Geometry: see drawing. Coordinates: mm, zero at the bounding-box minimum. A direction names the side the tool comes from. Coordinates: 2 decimals unless noted, no trailing zeros. Loops run counter-clockwise (first coordinate to the right, second up) from the corner with the lowest first, then second, coordinate; pieces in that order, holes last. Notation, with made-up numbers: (74.5, -29.5) - (131.5, -29.5) arc R23 ccw to (131.5, 5.5) - close; hole circle Ø2 at (38.5, 85). An arc over 180 degrees is marked (long way). Write each question's results on one line, items separated by ' | '. Start each with the question number.
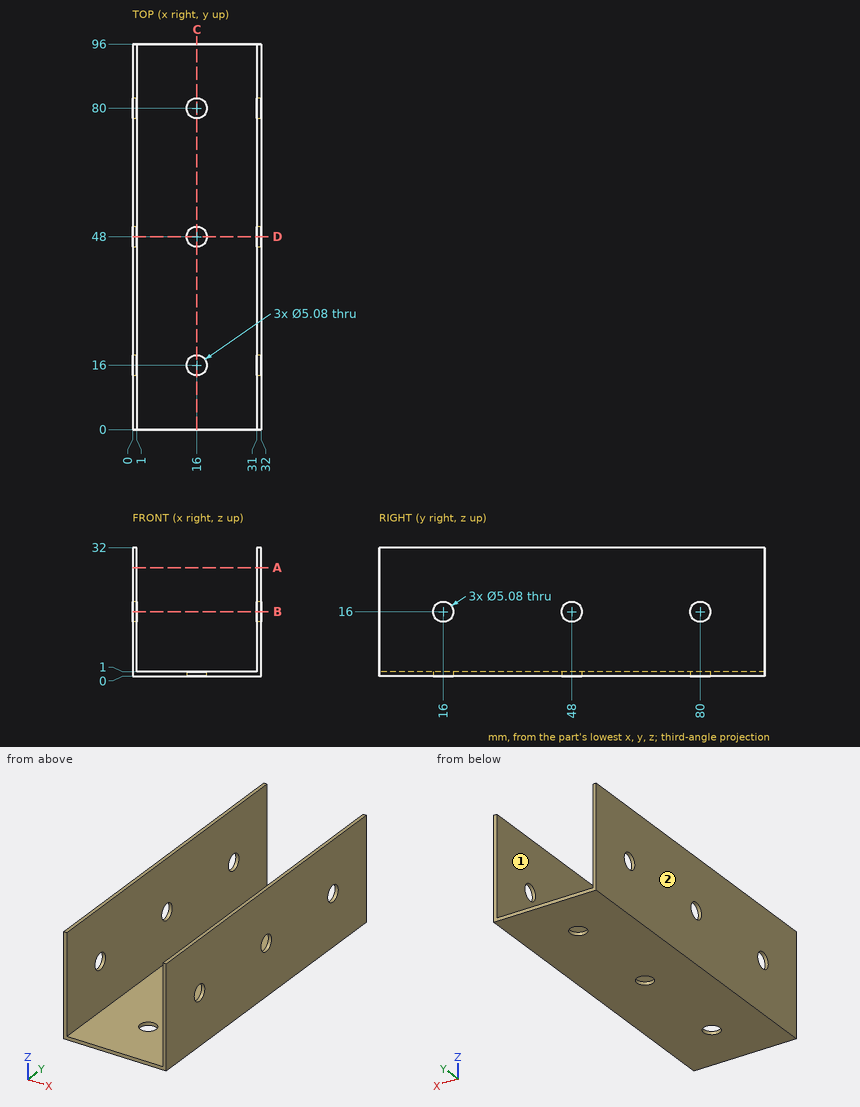
1) Material intervals for line 1 (Y direction, x = 16, z = 0.25); line 2 (X direction, y = 64.5, z = 8.5); line 3 (Z direction, x = 0.5, y = 16), sorted ascending. Write a range as [from, to].
2) Access query for the marked faces 1 and 2. Directions: +Z, -Z, +X, -X, +Y, -Y. A direction counts if a zero-diameter tool reaches every point of the face in a straight line with its end or side. Return the directions, or none.
3) Section query C-C on x = 16. Output: boundary loops of the cut face in (y, z).
4) Pin query (flat end, axial travel): pin 1 Ø10 at (x, y) = (5.5, 80) entering from +Z; pin 2 Ø15 at (x, y) = (18.5, 71) entering from +Z. Return the tip coordinate at first contact, or that it passes through.
5) Section query B-B on z = 16. Count the separate pieces of the cut face and the enclosed holes in it, and give its area (3 significant figures).
6) Section query D-D on y = 48. Output: boundary loops of the cut face in (x, z), and give its area (3 significant figures).
7) Section query A-A on z = 27. Output: boundary loops of the cut face in (x, y).
Returned:
1) line 1: y = [0, 13.46], [18.54, 45.46], [50.54, 77.46], [82.54, 96] | line 2: x = [0, 1], [31, 32] | line 3: z = [0, 13.46], [18.54, 32]
2) face 1: +Z, +Y, -Y | face 2: +Z, -Z, -X, +Y, -Y
3) outline: (0, 0) - (13.46, 0) - (13.46, 1) - (0, 1) - close; (18.54, 0) - (45.46, 0) - (45.46, 1) - (18.54, 1) - close; (50.54, 0) - (77.46, 0) - (77.46, 1) - (50.54, 1) - close; (82.54, 0) - (96, 0) - (96, 1) - (82.54, 1) - close
4) pin 1: stops at z = 32 | pin 2: stops at z = 1
5) separate pieces: 8 | enclosed holes: 0 | area: 162 mm²
6) outline: (0, 0) - (13.46, 0) - (13.46, 1) - (1, 1) - (1, 13.46) - (0, 13.46) - close; (0, 18.54) - (1, 18.54) - (1, 32) - (0, 32) - close; (18.54, 0) - (32, 0) - (32, 13.46) - (31, 13.46) - (31, 1) - (18.54, 1) - close; (31, 18.54) - (32, 18.54) - (32, 32) - (31, 32) - close | area: 78.8 mm²
7) outline: (0, 0) - (1, 0) - (1, 96) - (0, 96) - close; (31, 0) - (32, 0) - (32, 96) - (31, 96) - close
